Here's the drawing with two shaded views (mm, measured from the low corner). I have some questions. A direction names the side the tool comes from. Coordinates: 2 decimals unless noted, no trailing zeros. Order: outer loops, then holes, each group sorted by start corner. A loop starts at its lowest first (then second) coordinate and runs counter-clockwise, first axis right, second up. Notation, with made-up numbers: (20.25, -33) -> (79.25, -33) arc R24 ccw to (79.25, -11) -> close; hole circle Ø9 at (-11, -20). An arc over 180 degrees is marked (long way). Return JSON: item names as keys, results as strings. Group by question number.
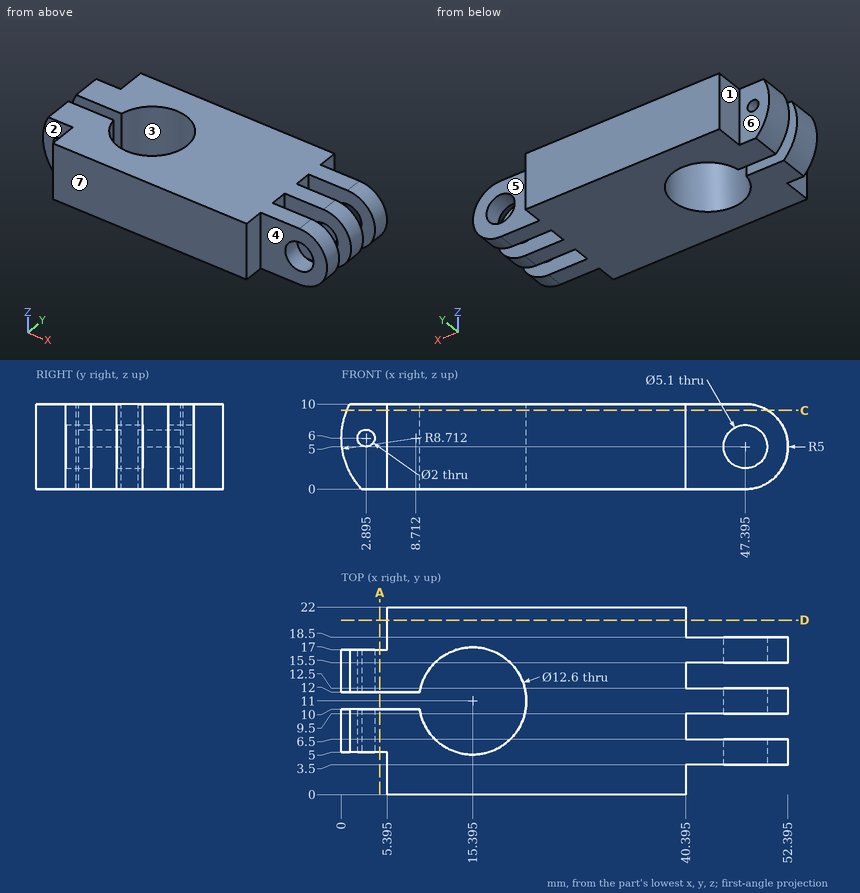
Q1. I want a section at A-A on x = 4.5. Please give me the cut outline in (y, z), and give its area (3 significant figures).
Q2. On a 3-axis mill with a long thin cutter (end or side, diameter ignored), from which of +Z, -Z, +X, -X, +Y, -Y can I reach the whole of each face in a straight line? I mean the marked faces 4, 5, 6 and 7. Say none if no direction works.
Q3. I need wall thicknesses on line 1 along Y through (x, z) = (48, 8.5); line 2 along Y through (x, z) = (9, 8.25); line 3 along X through (y, z) = (4.65, 5) (1 decimal). Which ranges of each line are inside material? Lowest first, please. Write a range as from..to.
Q4. We'd pull the mould along X, two halves only. Please class the marked faces 1, 2 and 3: pulls with the +X half, pulls with the -X half, needs draft (parallel to the pull), parting line crosses it, or undercut.
Q5. I want a section at D-D on y = 20.5. Please give me the cut outline in (x, z) (1 decimal), and give its area (3 significant figures).
Q6. I'm going to push flat-ended pins straight in: pin 1 Ø3 at (x, z) = (48, 3) entering from -Y; pin 2 Ø1.6 at (x, z) = (3, 3) entering from -Y; pin 3 Ø2.5 at (x, z) = (4, 5.5) entering from +Y; pin 4 Ø3 at (x, z) = (6.5, 7) entering from -Y. Where does each tip first touch, or does it pass through?
Q7. I want a section at C-C on z = 9.25. Please give me the cut outline in (x, y) (1 decimal), and give its area (3 significant figures).
Response values:
{
 "1": {"outline": "(5, 0) -> (10, 0) -> (10, 10) -> (5, 10) -> close; (12, 0) -> (17, 0) -> (17, 10) -> (12, 10) -> close", "area": "100 mm²"},
 "2": {"face 4": "+Z, -Z, +X, -Y", "face 5": "+Z, -Z, +X, +Y", "face 6": "+Z, -Z, -X, +Y", "face 7": "+Z, -Z, +X, -X, -Y"},
 "3": {"line 1": "y = 3.5..6.5, 9.5..12.5, 15.5..18.5", "line 2": "y = 0..10, 12..22", "line 3": "x = 5.4..44.8, 49.9..52.4"},
 "4": {"face 1": "pulls with the -X half", "face 2": "needs draft", "face 3": "undercut"},
 "5": {"outline": "(5.4, 0) -> (40.4, 0) -> (40.4, 10) -> (5.4, 10) -> close", "area": "350 mm²"},
 "6": {"pin 1": "stops at y = 3.5", "pin 2": "stops at y = 5", "pin 3": "stops at y = 17", "pin 4": "stops at y = 0"},
 "7": {"outline": "(0.6, 5) -> (5.4, 5) -> (5.4, 0) -> (40.4, 0) -> (40.4, 3.5) -> (50, 3.5) -> (50, 6.5) -> (40.4, 6.5) -> (40.4, 9.5) -> (50, 9.5) -> (50, 12.5) -> (40.4, 12.5) -> (40.4, 15.5) -> (50, 15.5) -> (50, 18.5) -> (40.4, 18.5) -> (40.4, 22) -> (5.4, 22) -> (5.4, 17) -> (0.6, 17) -> (0.6, 12) -> (9.2, 12) arc R6.3 cw (long way) to (9.2, 10) -> (0.6, 10) -> close", "area": "772 mm²"}
}
